from build123d import *

# Parameters (mm, degrees)
ESQUISSE1_R                  = 8
BOSS_EXTRU_1_DEPTH           = 2.4
ESQUISSE2_R                  = 2.5
BOSS_EXTRU_2_DEPTH           = 14
ESQUISSE3_R                  = 1
ENL_V_MAT_EXTRU_1_DEPTH      = 7
ESQUISSE4_R                  = 1.9
ENL_V_MAT_EXTRU_2_DEPTH      = 1.5
R_P_TITION_CIRCULAIRE2_COUNT = 4
CHANFREIN1_SIZE              = 0.5
ESQUISSE5_R                  = 1
ENL_V_MAT_EXTRU_3_DEPTH      = 1.6


with BuildPart() as part:
    # Esquisse1 → Boss.-Extru.1 (new body)
    with BuildSketch(Plane(origin=(0, 0, 0), x_dir=(1, 0, 0), z_dir=(0, 1, 0))):
        with Locations(Location((0, 0, 0), (0, 0, 270))):
            Circle(ESQUISSE1_R)
    extrude(amount=BOSS_EXTRU_1_DEPTH)

    # Esquisse2 → Boss.-Extru.2 (add)
    with BuildSketch(Plane(origin=(0, 2.4, 0), x_dir=(1, 0, 0), z_dir=(0, 1, 0))):
        with Locations(Location((0, 0, 0), (0, 0, 270))):
            Circle(ESQUISSE2_R)
    extrude(amount=BOSS_EXTRU_2_DEPTH)

    # Esquisse3 → Enlèv. mat.-Extru.1 (cut)
    with BuildSketch(Plane(origin=(0, 2.4, 0), x_dir=(1, 0, 0), z_dir=(0, 1, 0))):
        with Locations(Location((4.5, 0, 0), (0, 0, 270))):
            Circle(ESQUISSE3_R)
    enl_v_mat_extru_1 = extrude(amount=-ENL_V_MAT_EXTRU_1_DEPTH, mode=Mode.SUBTRACT)

    # Esquisse4 → Enlèv. mat.-Extru.2 (cut)
    with BuildSketch(Plane(origin=(0, 2.4, 0), x_dir=(1, 0, 0), z_dir=(0, 1, 0))):
        with Locations(Location((4.5, 0, 0), (0, 0, 270))):
            Circle(ESQUISSE4_R)
    enl_v_mat_extru_2 = extrude(amount=-ENL_V_MAT_EXTRU_2_DEPTH, mode=Mode.SUBTRACT)

    # Répétition circulaire2: Enlèv. mat.-Extru.1, Enlèv. mat.-Extru.2 ×4 about axis
    r_p_tition_circulaire2_axis = Axis((0, 0, 0), (0, 1, 0))
    add([enl_v_mat_extru_1.rotate(r_p_tition_circulaire2_axis, i * 360 / R_P_TITION_CIRCULAIRE2_COUNT) for i in range(1, R_P_TITION_CIRCULAIRE2_COUNT)], mode=Mode.SUBTRACT)
    add([enl_v_mat_extru_2.rotate(r_p_tition_circulaire2_axis, i * 360 / R_P_TITION_CIRCULAIRE2_COUNT) for i in range(1, R_P_TITION_CIRCULAIRE2_COUNT)], mode=Mode.SUBTRACT)

    # Chanfrein1
    chanfrein1_edges = [part.edges().sort_by_distance(p)[0] for p in [
        (0, 16.4, -2.5),
    ]]
    chamfer(chanfrein1_edges, length=CHANFREIN1_SIZE)

    # Esquisse5 → Enlèv. mat.-Extru.3 (cut)
    with BuildSketch(Plane.XZ):
        with Locations(Location((0, 0, 0), (0, 0, 270))):
            Circle(ESQUISSE5_R)
    extrude(amount=-ENL_V_MAT_EXTRU_3_DEPTH, mode=Mode.SUBTRACT)


solid = part.part
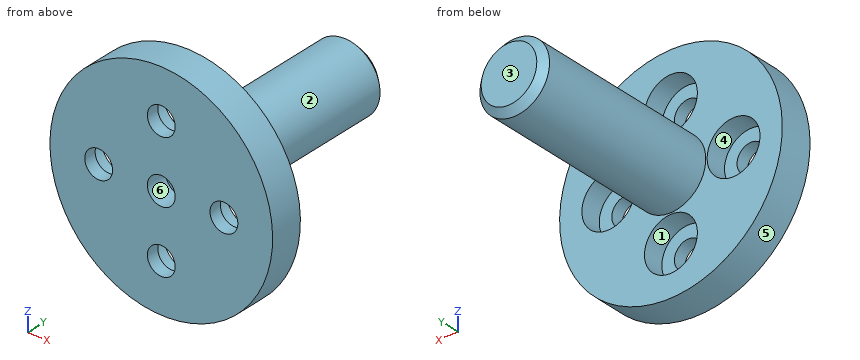
The model under review builds one solid part; all positions refer to its coordinate system, in mm. Face numbers are marked on the shaded views. A direction names the side the tool comes from. Coordinates: 2 decimals unless noted, no trailing zeros. Order: outer loops, then holes, each group sorted by start corner. A loop starts at its lowest first (then second) coordinate and runs counter-clockwise, first axis right, second up. Notation, with made-up numbers: (39, -22) -> (57, -22) arc R11 ccw to (57, -6) -> close; hole circle Ø5 at (59.25, 78.5). An arc over 180 degrees is marked (long way). Answer in a Markdown table with one row per item.
(1) Machinability: for the marked faces 4, 5 and 6, which of the approach directions +Z, -Z, +X, -X, +Y, -Y give a long, thin tool a straight path to every point of the face, cutting with its end or side? Answer none if there is none.
Answers:
| item | result |
|---|---|
| face 4 | +Y |
| face 5 | +Y, -Y |
| face 6 | -Y |
(2) Consider section A-A (x = 0). State how many separate pieces and enclosed holes the cut face has, plus the area to 4 significant figures.
Answers:
| item | result |
|---|---|
| separate pieces | 3 |
| enclosed holes | 0 |
| area | 89.95 mm² |
(3) Insertion check: pin 1 (5 mm diameter, centred on y = 10, z = 0.5, fed in from +X); pin 2 (2.5 mm diameter, centred on x = 4.5, z = 0, fed in from +Y); pin 3 (5 mm diameter, centred on x = 0.5, z = -3.5, fed in from +Y); pin 4 (1 mm diameter, centred on y = 7.5, z = 2, fed in from -X). Each pin has a flat end and moves straight along its axis. Give the tip position at first contact, or say it passes through.
Answers:
| item | result |
|---|---|
| pin 1 | x = 2.5 |
| pin 2 | y = 0.9 |
| pin 3 | y = 16.4 |
| pin 4 | x = -2 |
(4) Wall thickness on line 1 along X through (y, z) = (0.4, 0); line 2 along Y through (x, z) = (-3, 4); line 3 along X through (y, z) = (2.5, 0): over which ranges is each line inside the solid? List them lowest first.
Answers:
| item | result |
|---|---|
| line 1 | -8 to -5.5, -3.5 to -1, 1 to 3.5, 5.5 to 8 |
| line 2 | 0 to 2.4 |
| line 3 | -2.5 to 2.5 |
(5) The part is to be moulded in two halves that separate along X. For the marked faces 1, 2 and 3, say which applies: +X half, -X half, draft (parallel to the pull), parting line (faces both ways), or undercut.
Answers:
| item | result |
|---|---|
| face 1 | undercut |
| face 2 | parting line |
| face 3 | draft |
(6) Consider section D-D (z = 4.75). Write out the cut boundary in (x, y), plus the area to 3 significant figures.
Answers:
| item | result |
|---|---|
| outline | (-6.44, 0) -> (-0.97, 0) -> (-0.97, 0.9) -> (-1.88, 0.9) -> (-1.88, 2.4) -> (-6.44, 2.4) -> close; (0.97, 0) -> (6.44, 0) -> (6.44, 2.4) -> (1.88, 2.4) -> (1.88, 0.9) -> (0.97, 0.9) -> close |
| area | 23.5 mm² |
(7) Consider section C-C (x = -4.5). Write out the cut boundary in (y, z).
Answers:
| item | result |
|---|---|
| outline | (0, -6.61) -> (2.4, -6.61) -> (2.4, -1.9) -> (0.9, -1.9) -> (0.9, -1) -> (0, -1) -> close; (0, 1) -> (0.9, 1) -> (0.9, 1.9) -> (2.4, 1.9) -> (2.4, 6.61) -> (0, 6.61) -> close |
